Geometry: final body of the model. Coordinates: model frame, mm. Round coordinates to 2 decimals unless told otherwise and drop trailing zeros. Loops run counter-clockwise (first coordinate to the right, second up) from the corner with the lowest first, then second, coordinate; pieces in that order, holes last. Notation, with made-up numbers: (57, 77) - (104, 77) arc R11 cw to (104, 90) - close; hole circle Ø6 at (24.25, 33). An arc over 180 degrees is marked (long way). Write item = value, one per line. Start each with the question number.
Item 1: Line query: line 1 (X direction, y = -4, z = 7.75); line 2 (X direction, y = 11, z = 3.25); line 3 (Y direction, x = 24, z = 5.5). Output: solid intervals per line, ascending. Write a range as from..to.
Item 2: Draft query along Y for faces 1 (the flat face through (-6, -7, 8)), 2 (the flat face through (0, 7, 0)). Return one class per face: pulls with the +Y half, pulls with the -Y half, needs draft (parallel to the pull), parting line crosses it, or undercut.
Item 3: First-contact query: pin 1 (4 mm diameter, centred on y = 14.5, z = 5.5, fed in from +X); pin 2 (0.9 mm diameter, centred on x = 0.5, z = 3.5, fed in from +Y); pin 3 (14.5 mm diameter, centred on x = 0.5, y = -14, fed in from -Z); pin 4 (2.5 mm diameter, centred on y = 23, z = 4.5, fed in from +X). Flat tips, straight axial feed; report the tip coordinate or a pass-through.
Item 4: Section B-B (z = 2.75). Count the separate pieces of the cut face and the enclosed holes in it, plus the area to 3 significant figures.
Item 5: Section A-A (y = 0). Return loops of the section in (x, z), plus the area to 3 significant figures.
from build123d import *

# Parameters (mm, degrees)
F1_R     = 28.434676
F2_DEPTH = 10
F3_DEPTH = 8


with BuildPart() as f2:
    # F1 (on Top) → F2 (new body)
    with BuildSketch(Plane.XY):
        Circle(F1_R)
    extrude(amount=F2_DEPTH)

    # F0 (on Top) → F3 (cut)
    with BuildSketch(Plane.XY):
        Polygon((-17.364958, 7.356322), (-17.232909, 7.654685), (-16.881704, 8.45762), (-15.524421, 10.731926), (-13.289539, 13.42287), (-10.598709, 15.657751), (-8.324306, 17.015878), (-7.521533, 17.367132), (-7.223008, 17.499197), (-4.087684, 18.495686), (-3.761253, 18.562368), (-3.761253, 26.192278), (-4.083303, 26.146526), (-7.216843, 25.450184), (-7.521533, 25.355921), (-8.310191, 25.121806), (-10.614544, 24.219579), (-13.511356, 22.718842), (-16.184583, 20.883562), (-18.606935, 18.740996), (-20.749388, 16.318725), (-22.584635, 13.645466), (-24.085421, 10.747988), (-24.987648, 8.443342), (-25.22178, 7.654685), (-25.315961, 7.350319), (-26.012222, 4.216617), (-26.05799, 3.894567), (-18.428258, 3.894567), (-18.36135, 4.220998), align=None)
        Polygon((16.879968, 8.45762), (17.232033, 7.654685), (17.363124, 7.356322), (18.360425, 4.220998), (18.427431, 3.894567), (26.05799, 3.894567), (26.011265, 4.216617), (25.314923, 7.350319), (25.221634, 7.654685), (24.986707, 8.443342), (24.08448, 10.747988), (22.583743, 13.645466), (20.748625, 16.318725), (18.606059, 18.740996), (16.183626, 20.883562), (13.510529, 22.718842), (10.613701, 24.219579), (8.309379, 25.121806), (7.521533, 25.355921), (7.216031, 25.450184), (4.081519, 26.146526), (3.76028, 26.192278), (3.76028, 18.562368), (4.085899, 18.495686), (7.222034, 17.499197), (7.521533, 17.367132), (8.323332, 17.015878), (10.597801, 15.657751), (13.288582, 13.42287), (15.52249, 10.731926), align=None)
        Polygon((-8.28196, -24.853474), (2.331578, -3.625992), (14.566724, -3.625992), (14.643302, -3.325033), (15.042903, -0.731111), (15.042903, 0.133314), (15.042903, 1.074317), (14.643302, 3.595231), (14.566724, 3.895378), (-14.56674, 3.895378), (-14.64421, 3.595231), (-15.042936, 0.999361), (-15.042936, 0.133314), (-15.042936, -0.805904), (-14.64421, -3.325033), (-14.56674, -3.625992), (-6.08407, -3.625992), (-11.600391, -14.64997), (-11.860075, -14.446648), (-13.086218, -13.35429), (-14.219915, -12.161601), (-14.432955, -11.908975), (-14.665318, -11.630827), (-16.659027, -8.592378), (-16.823605, -8.264811), (-16.859704, -8.191803), (-17.202116, -7.460416), (-17.232909, -7.388219), (-17.364958, -7.088882), (-18.36135, -3.951774), (-18.428258, -3.625992), (-26.05799, -3.625992), (-26.012222, -3.947393), (-25.316853, -7.082717), (-25.222672, -7.388219), (-24.986756, -8.185637), (-23.372433, -11.967073), (-21.228228, -15.431619), (-20.726496, -16.071517), (-20.519653, -16.338226), (-19.423791, -17.618071), (-18.248689, -18.817801), (-18.001351, -19.0458), (-17.76808, -19.266724), (-15.273546, -21.293855), (-15.009482, -21.478697), (-14.498079, -21.835208), (-11.784357, -23.401118), (-8.885825, -24.652781), align=None)
        Polygon((17.363124, -7.088882), (17.232033, -7.388219), (16.879968, -8.190018), (15.52249, -10.463659), (13.288582, -13.154473), (10.597801, -15.389355), (8.323332, -16.746654), (7.521533, -17.098735), (7.222034, -17.229908), (4.085899, -18.2263), (3.76028, -18.293192), (3.728643, -18.299373), (3.407404, -18.355704), (3.376578, -18.360101), (-0.543186, -26.183484), (-0.497271, -26.185237), (-0.124926, -26.192278), (0, -26.192278), (0.940192, -26.192278), (3.453156, -25.967833), (3.76028, -25.923816), (4.081519, -25.877156), (7.216031, -25.181787), (7.521533, -25.087606), (8.309379, -24.852582), (10.613701, -23.950371), (13.510529, -22.449585), (16.183626, -20.614338), (18.606059, -18.471885), (20.748625, -16.049533), (22.583743, -13.376306), (24.08448, -10.48037), (24.986707, -8.175903), (25.221634, -7.388219), (25.314923, -7.082717), (26.011265, -3.948367), (26.05799, -3.626966), (18.427431, -3.626966), (18.360425, -3.952747), align=None)
    extrude(amount=F3_DEPTH, mode=Mode.SUBTRACT)


solid = f2.part
Taken from the geometry:
q1.line_1 = -28.15..-26, -18.35..-6.27, 2.14..18.35, 26..28.15
q1.line_2 = -26.22..-23.95, -15.3..15.3, 23.95..26.22
q1.line_3 = -15.25..-10.64, -3.63..3.89, 10.91..15.25
q2.face_1 = undercut
q2.face_2 = needs draft
q3.pin_1 = 25.54
q3.pin_2 = 28.43
q3.pin_3 = 0
q3.pin_4 = 18.32
q4.separate_pieces = 1
q4.enclosed_holes = 4
q4.area = 1,370 mm^2
q5.outline = (-28.43, 0) - (-15.04, 0) - (-15.04, 8) - (15.04, 8) - (15.04, 0) - (28.43, 0) - (28.43, 10) - (-28.43, 10) - close
q5.area = 328 mm^2
